Job drawing, mm, ordinate dimensions from the low corner. One solid piece. A direction names the side the tool comes from. Give positions to 0.01 mm unless a question says otherwise; leave off trailing zeros. Order: outer loops, then holes, each group sorted by start corner. A loop starts at its lowest first (then second) coordinate and runs counter-clockwise, first axis right, second up. Notation, with made-up numbers: M 5,24.25 L 13,24.25 A10 cw 13,43.25 Z; hole C 20,33 d1. An arc over 180 degrees is marked long. One line per item, written item: value. Start each with the question number.
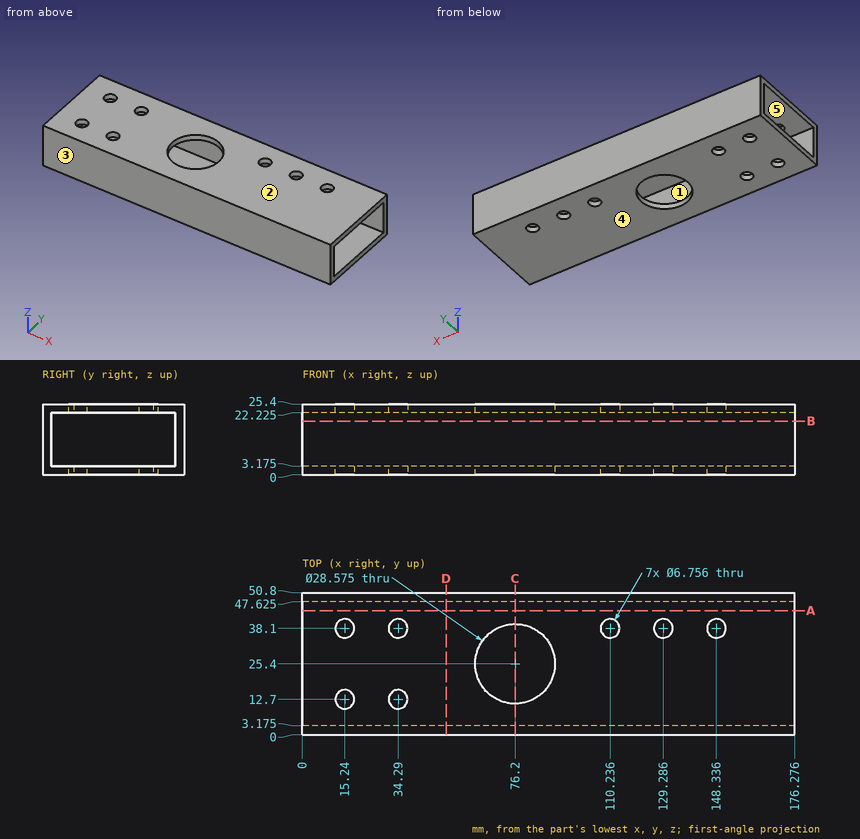
1) Drop a flat-ended pin along its axis: P1, Ø9, axis at x = 110.236, y = 38.1, coming from the +Z side. Give the stop position or say it passes through.
2) Slice it at A-A (y = 44.5). List the corners of the cut face in (x, z) (1 decimal), plus the area to 3 significant figures.
3) Pull direction Y, two halves, no side cores. Call the marked faces 3, 4 and 5: pulls with the +Y half, pulls with the -Y half, needs draft (parallel to the pull), parting line crosses it, or undercut.
4) Drill centre lines: line 1 (Y direction, x = 34.29, z = 24.05); line 2 (Y direction, x = 94, z = 12) (1 decimal); line 3 (Z direction, x = 55.5, y = 40.5) (1 decimal). Where is each one in solid material? Low to high.
5) Slice it at B-B (z = 19.25). List the corners of the cut face in (x, y) (1 decimal), plus the area to 3 significant figures.
6) Slice it at C-C (x = 76.2). List the corners of the cut face in (y, z) (1 decimal), plus the area to 3 significant figures.
7) Tool access for the marked faces 1 and 2: list every direction of +Z, -Z, +X, -X, +Y, -Y with a clear straight run to the whole face (end or side of a thin tool).
8) Slice it at D-D (x = 51.5). List the corners of the cut face in (y, z) (1 decimal).
Results list:
1. P1: stops at z = 25.4
2. outline: M 0,0 L 176.3,0 L 176.3,3.2 L 0,3.2 Z; M 0,22.2 L 176.3,22.2 L 176.3,25.4 L 0,25.4 Z
2. area: 1,120 mm²
3. face 3: pulls with the -Y half
3. face 4: needs draft
3. face 5: undercut
4. line 1: y = 0 to 9.32, 16.08 to 34.72, 41.48 to 50.8
4. line 2: y = 0 to 3.2, 47.6 to 50.8
4. line 3: z = 0 to 3.2, 22.2 to 25.4
5. outline: M 0,0 L 176.3,0 L 176.3,3.2 L 0,3.2 Z; M 0,47.6 L 176.3,47.6 L 176.3,50.8 L 0,50.8 Z
5. area: 1,120 mm²
6. outline: M 0,0 L 11.1,0 L 11.1,3.2 L 3.2,3.2 L 3.2,22.2 L 11.1,22.2 L 11.1,25.4 L 0,25.4 Z; M 39.7,0 L 50.8,0 L 50.8,25.4 L 39.7,25.4 L 39.7,22.2 L 47.6,22.2 L 47.6,3.2 L 39.7,3.2 Z
6. area: 262 mm²
7. face 1: +X, -X
7. face 2: +Z, +X, -X, +Y, -Y
8. outline: M 0,0 L 50.8,0 L 50.8,25.4 L 0,25.4 Z; hole M 3.2,3.2 L 47.6,3.2 L 47.6,22.2 L 3.2,22.2 Z
